The listing builds one solid part. Answer for the finished solid, in the listing's coordinates (mm). A direction names the side the tool comes from. Give positions to 0.01 mm unless a question says otherwise; leave off trailing zeros. Write each loop counter-clockwise with the first axis right and the second up, starting at its lowest first coordinate (ties: lowest second). Pieces come first, ordered by that corner, then holes.
```python
from build123d import *

# Parameters (mm, degrees)
PAD_DEPTH       = 3.6
SKETCH001_W     = 7.9
SKETCH001_H     = 3
PAD001_DEPTH    = 0.5
SKETCH002_W     = 0.3
SKETCH002_H     = 0.6
PAD002_DEPTH    = 0.3
SKETCH003_W     = 0.25
SKETCH003_H     = 2.2
POCKET_DEPTH    = 3.501
POCKET001_DEPTH = 0.2
SKETCH014_W     = 3.5
SKETCH014_H     = 0.8
POCKET002_DEPTH = 0.2
SKETCH015_W     = 1.5
SKETCH015_H     = 1.5
PAD008_DEPTH    = 2.2
POCKET003_DEPTH = 4.251


with BuildPart() as part:
    # Sketch (on DatumPlane) → Pad (new body)
    with BuildSketch(Plane.XZ.offset(-0.15)):
        Polygon((-1.75, 0.8), (-1.75, 2.5), (-2, 2.5), (-1.8, 3.5), (6.8, 3.5), (7, 2.5), (6.75, 2.5), (6.75, 0.8), align=None)
    extrude(amount=PAD_DEPTH)

    # Sketch001 (on Face8 of Pad) → Pad001 (join)
    with BuildSketch(Plane(origin=(0, 0.15, 0.8), x_dir=(1, 0, 0), z_dir=(0, 0, -1))):
        with Locations((2.5, 1.8)):
            Rectangle(SKETCH001_W, SKETCH001_H)
    extrude(amount=PAD001_DEPTH)

    # Sketch002 (on Face15 of Pad001) → Pad002 (join)
    with BuildSketch(Plane(origin=(0, 0.15, 0.3), x_dir=(1, 0, 0), z_dir=(0, 0, -1))):
        with Locations((-0.85, 2.8)):
            Rectangle(SKETCH002_W, SKETCH002_H)
        with Locations((-0.85, 0.8)):
            Rectangle(SKETCH002_W, SKETCH002_H)
        with Locations((5.85, 2.8)):
            Rectangle(SKETCH002_W, SKETCH002_H)
        with Locations((5.85, 0.8)):
            Rectangle(SKETCH002_W, SKETCH002_H)
    extrude(amount=PAD002_DEPTH)

    # Sketch003 (on Face12 of Pad002) → Pocket (cut, through all)
    with BuildSketch(Plane(origin=(0, 0.15, 3.5), x_dir=(-1, 0, 0), z_dir=(0, 0, 1))):
        with Locations((1.875, 1.8)):
            Rectangle(SKETCH003_W, SKETCH003_H)
        with Locations((-6.875, 1.8)):
            Rectangle(SKETCH003_W, SKETCH003_H)
    extrude(amount=-POCKET_DEPTH, mode=Mode.SUBTRACT)

    # Sketch004 (on Face7 of Pocket) → Pocket001 (cut)
    with BuildSketch(Plane(origin=(0, 0.15, 3.5), x_dir=(-1, 0, 0), z_dir=(0, 0, 1))):
        Polygon((-5.5, 3.6), (-5.5, 3.25), (-6.5, 3.25), (-6.5, 2.9), (-6.75, 2.9), (-6.75, 0.7), (-6.5, 0.7), (-6.5, 0.35), (-5.5, 0.35), (-5.5, 0), (0.5, 0), (0.5, 0.35), (1.5, 0.35), (1.5, 0.7), (1.75, 0.7), (1.75, 2.9), (1.5, 2.9), (1.5, 3.25), (0.5, 3.25), (0.5, 3.6), align=None)
    extrude(amount=-POCKET001_DEPTH, mode=Mode.SUBTRACT)

    # Sketch014 (on Face20 of Pocket001) → Pocket002 (cut)
    with BuildSketch(Plane.XZ.offset(3.45)):
        with Locations((2.5, 2.9)):
            Rectangle(SKETCH014_W, SKETCH014_H)
    extrude(amount=-POCKET002_DEPTH, mode=Mode.SUBTRACT)

    # Sketch015 (on Face40 of Pocket002) → Pad008 (join)
    with BuildSketch(Plane.XZ.offset(3.25)):
        with Locations((1.5, 2.55)):
            Rectangle(SKETCH015_W, SKETCH015_H)
    extrude(amount=PAD008_DEPTH)

    # Sketch016 (on Face50 of Pad008) → Pocket003 (cut, through all)
    with BuildSketch(Plane(origin=(2.25, 0.15, 0), x_dir=(0, 0, 1), z_dir=(1, 0, 0))):
        Polygon((1.8, 4.6), (1.8, 3.6), (2.5, 3.6), align=None)
    extrude(amount=-POCKET003_DEPTH, mode=Mode.SUBTRACT)


solid = part.part
```
Item 1: A cutting plane is placed at C-C, the plane x = 1.75. Give the vertices of the cut face in (y, z).
Conclusion:
outline: (-5.45, 1.8) - (-4.45, 1.8) - (-3.45, 2.5) - (-3.45, 0.8) - (-3.15, 0.8) - (-3.15, 0.3) - (-0.15, 0.3) - (-0.15, 0.8) - (0.15, 0.8) - (0.15, 3.3) - (-5.45, 3.3) - close
Item 2: Which of the six approach directions +Z, -Z, +X, -X, +Y, -Y give full straight-line access (tool end or side, diameter ignored) to faces 1 (the face through (1, -5.45, 3)), 2 (the face through (1, -5, 1.8)), 3 (the face through (1.51, -3.943, 2.155))?
Conclusion:
face 1: +Z, -Z, +X, -X, -Y
face 2: -Z, +X, -X, -Y
face 3: -Z, +X, -X
Item 3: A cutting plane is placed at A-A, the plane y = -2.85. Give the vertices of the cut face in (x, z), plus the area to 3 significant figures.
Conclusion:
outline: (-2, 2.5) - (-1.75, 2.5) - (-1.75, 0.8) - (-1.45, 0.8) - (-1.45, 0.3) - (-1, 0.3) - (-1, 0) - (-0.7, 0) - (-0.7, 0.3) - (5.7, 0.3) - (5.7, 0) - (6, 0) - (6, 0.3) - (6.45, 0.3) - (6.45, 0.8) - (6.75, 0.8) - (6.75, 2.5) - (7, 2.5) - (6.8, 3.5) - (6.5, 3.5) - (6.5, 3.3) - (-1.5, 3.3) - (-1.5, 3.5) - (-1.8, 3.5) - close
area: 25.8 mm2
Item 4: Each of these flat-tipped pins is pushed along its axis until it touches: P1, Ø1.6, axis at y = -4, z = 2.5, coming from the +X side; P2, Ø3, axis at x = 3.5, y = -3.5, coming from the -Z side; P3, Ø1.2, axis at y = -4.5, z = 2.5, coming from the -X side. Where does it stop, or does it pass through?
Conclusion:
P1: stops at x = 7
P2: stops at z = 0.3
P3: stops at x = 0.75
Item 5: A cutting plane is placed at D-D, the plane z = 1.2. Give the vertices of the cut face in (x, y), plus the area to 3 significant figures.
Conclusion:
outline: (-1.75, -3.45) - (6.75, -3.45) - (6.75, 0.15) - (-1.75, 0.15) - close
area: 30.6 mm2
Item 6: Consider probe 1 along X at (y, z) = (-2.65, 0.2); probe 2 along Y at (x, z) = (3.5, 3.1); probe 3 along X at (y, z) = (-3.1, 2.1). Determine where each line is inside the solid, lowest interval first.
Conclusion:
probe 1: x = -1 to -0.7, 5.7 to 6
probe 2: y = -3.25 to 0.15
probe 3: x = -1.75 to 6.75
Item 7: Determine the mould class of faces 4 (the face through (3, 0.15, 2)), 5 (the face through (0.75, -4, 3)), 6 (the face through (2, -2, 3.3)) for opening direction Y: pulls with the +Y half, pulls with the -Y half, needs draft (parallel to the pull), parting line crosses it, or undercut.
Conclusion:
face 4: pulls with the +Y half
face 5: needs draft
face 6: undercut
Item 8: A cutting plane is placed at B-B, the plane z = 2.05. Give the vertices of the cut face in (x, y), plus the area to 3 significant figures.
Conclusion:
outline: (-1.75, -3.45) - (6.75, -3.45) - (6.75, 0.15) - (-1.75, 0.15) - close; (0.75, -5.45) - (2.25, -5.45) - (2.25, -4.09) - (0.75, -4.09) - close
area: 32.6 mm2
